```python
from build123d import *

# Parameters (mm, degrees)
SKETCH1_W               = 15
SKETCH1_H               = 15
BOSS_EXTRUDE1_DEPTH     = 5
SKETCH2_W               = 3
SKETCH2_H               = 15
BOSS_EXTRUDE2_DEPTH     = 5
CUT_EXTRUDE1_DEPTH      = 18
SKETCH4_R               = 1.5
CUT_EXTRUDE2_DEPTH      = 13
CUT_EXTRUDE2_DEPTH_BACK = 4


with BuildPart() as part:
    # Sketch1 → Boss-Extrude1 (new body)
    with BuildSketch(Plane.XY):
        with Locations((-7.5, -7.5)):
            Rectangle(SKETCH1_W, SKETCH1_H)
    extrude(amount=BOSS_EXTRUDE1_DEPTH)

    # Sketch2 → Boss-Extrude2 (add)
    with BuildSketch(Plane.XY.offset(5)):
        with Locations((-1.5, -7.5)):
            Rectangle(SKETCH2_W, SKETCH2_H)
        with Locations((-13.5, -7.5)):
            Rectangle(SKETCH2_W, SKETCH2_H)
    extrude(amount=BOSS_EXTRUDE2_DEPTH)

    # Sketch3 → Cut-Extrude1 (cut)
    with BuildSketch(Plane(origin=(0, 0, 0), x_dir=(0, 0, -1), z_dir=(1, 0, 0))):
        with BuildLine():
            Line((-7.733661886, 0), (-10, 0))
            Line((-10, 0), (-10, -15))
            Line((-10, -15), (-7.733661886, -15))
            ThreePointArc((-7.733661886, -15), (-9.654849758, -7.5), (-7.733661886, 0))
        make_face()
    extrude(amount=-CUT_EXTRUDE1_DEPTH, mode=Mode.SUBTRACT)

    # Sketch4 → Cut-Extrude2 (cut, two sides)
    with BuildSketch(Plane(origin=(-12, 0, 0), x_dir=(0, 0, -1), z_dir=(1, 0, 0))) as cut_extrude2_sk:
        with Locations((-7.041389116, -7.762480296)):
            Circle(SKETCH4_R)
    extrude(amount=CUT_EXTRUDE2_DEPTH, mode=Mode.SUBTRACT)
    extrude(cut_extrude2_sk.sketch, amount=-CUT_EXTRUDE2_DEPTH_BACK, mode=Mode.SUBTRACT)


solid = part.part
```
CAD build for the part. Positions are in the model's coordinates, mm. A direction names the side the tool comes from. Coordinates: 2 decimals unless noted, no trailing zeros. Order: outer loops, then holes, each group sorted by start corner. A loop starts at its lowest first (then second) coordinate and runs counter-clockwise, first axis right, second up.
(1) Saw through at B-B, the plane y = -6.75. Write the cut outline in (x, z), and give its area (3 significant figures).
Solution:
outline: (-15, 0) - (0, 0) - (0, 5.93) - (-3, 5.93) - (-3, 5) - (-12, 5) - (-12, 5.93) - (-15, 5.93) - close; (-15, 8.15) - (-12, 8.15) - (-12, 9.64) - (-15, 9.64) - close; (-3, 8.15) - (0, 8.15) - (0, 9.64) - (-3, 9.64) - close
area: 89.5 mm2
(2) Drill centre lines: L1, parallel to X at y = -5.5, z = 8.5; L2, parallel to Y at x = -14, z = 7; L3, parallel to Z at x = -9.75, y = -4.5. Where is each one in solid material? Low to high.
Solution:
L1: x = -15 to -12, -3 to 0
L2: y = -15 to -9.26, -6.26 to 0
L3: z = 0 to 5
(3) Saw through at A-A, the plane z = 5.75. Write the cut outline in (x, y).
Solution:
outline: (-15, -15) - (-12, -15) - (-12, -8.53) - (-15, -8.53) - close; (-15, -7) - (-12, -7) - (-12, 0) - (-15, 0) - close; (-3, -15) - (0, -15) - (0, -8.53) - (-3, -8.53) - close; (-3, -7) - (0, -7) - (0, 0) - (-3, 0) - close
(4) Mould opens along Z. For faces 1 (the face through (-13.479, -6.275, 7.237)), 2 (the face through (-8, -15, 3)), 3 (the face through (-13.479, -7.61, 9.654)) say: released by +Z, released by -Z, zero draft, split by the parting line, or undercut.
Solution:
face 1: undercut
face 2: zero draft
face 3: released by +Z
(5) Pin check, flat tips, straight feed: pin 1 Ø4 at (y, z) = (-7.76, 7.04) entering from -X; pin 2 Ø4.5 at (x, y) = (-9, -6) entering from +Z. Stop position of each tip, or through.
Solution:
pin 1: stops at x = -15
pin 2: stops at z = 5
(6) Saw through at C-C, the plane y = -3.5. Write the cut outline in (x, z), and give its area (3 significant figures).
Solution:
outline: (-15, 0) - (0, 0) - (0, 9.13) - (-3, 9.13) - (-3, 5) - (-12, 5) - (-12, 9.13) - (-15, 9.13) - close
area: 99.8 mm2
(7) Which spindle directions (+Z, -Z, +X, -X, +Y, -Y) get a long thin tool onto all of the face, cutting with end or side? Do faces 4 (the face through (-12, -6, 7)), 5 (the face through (-1.521, -6.275, 7.237)). Say none if no direction does.
Solution:
face 4: +Z, +Y, -Y
face 5: +X, -X
(8) Saw through at D-D, the plane x = -13.5. Write the cut outline in (y, z).
Solution:
outline: (-15, 0) - (0, 0) - (0, 7.73) arc R15.6 ccw to (-15, 7.73) - close; hole circle Ø3 at (-7.76, 7.04)
